Source: CAD feature listing. Evaluate the final solid. Frame: model axes, mm. Face numbers are marked on the shaded views. Coordinates: 2 decimals unless noted, no trailing zeros. Loops run counter-clockwise (first coordinate to the right, second up) from the corner with the lowest first, then second, coordinate; pieces in that order, holes last. Notation, with made-up numbers: (75, -30.5) - (86, -30.5) arc R20 cw to (86, -24.5) - close; hole circle Ø2 at (88, 46). An arc over 180 degrees is marked (long way). Write item = value, one per line. Start each with the question number.
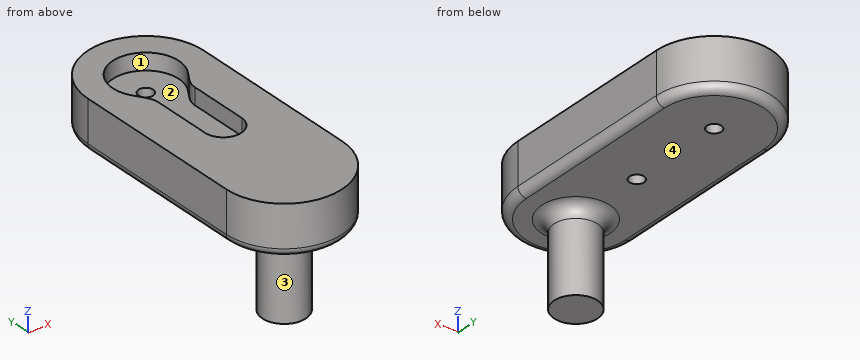
from build123d import *

# Parameters (mm, degrees)
PAD_DEPTH       = 12
POCKET_DEPTH    = 4
SKETCH002_R     = 5.25
PAD001_DEPTH    = 20
SKETCH003_R     = 1.75
POCKET001_DEPTH = 28.001
FILLET_R        = 3
FILLET001_R     = 2
FILLET002_R     = 5


with BuildPart() as part:
    # Sketch001 → Pad (new body)
    with BuildSketch(Plane.XY):
        with BuildLine():
            ThreePointArc((14, 0), (0, 14), (-14, 0))
            Line((-14, 0), (-14, -42))
            ThreePointArc((-14, -42), (0, -56), (14, -42))
            Line((14, -42), (14, 0))
        make_face()
    extrude(amount=PAD_DEPTH)

    # Sketch (on Face6 of Pad) → Pocket (cut)
    with BuildSketch(Plane.XY.offset(12)):
        with BuildLine():
            ThreePointArc((6.614378, -4.5), (0, 8), (-6.614378, -4.5))
            Line((-6.614378, -4.5), (-4.395452, -8))
            Line((-4.395452, -8), (-4.395452, -23.7))
            ThreePointArc((-4.395452, -23.7), (0, -27.9), (4.395452, -23.7))
            Line((4.395452, -8), (4.395452, -23.7))
            Line((6.614378, -4.5), (4.395452, -8))
        make_face()
    extrude(amount=-POCKET_DEPTH, mode=Mode.SUBTRACT)

    # Sketch002 (on Face4 of Pocket) → Pad001 (join)
    with BuildSketch(Plane(origin=(0, 0, 0), x_dir=(1, 0, 0), z_dir=(0, 0, -1))):
        with Locations((0, 42)):
            Circle(SKETCH002_R)
    extrude(amount=PAD001_DEPTH)

    # Sketch003 (on Face15 of Pad001) → Pocket001 (cut, through all)
    with BuildSketch(Plane.XY.offset(8)):
        Circle(SKETCH003_R)
        with Locations((0, -23.5)):
            Circle(SKETCH003_R)
    extrude(amount=-POCKET001_DEPTH, mode=Mode.SUBTRACT)

    # Fillet
    fillet_edges = [part.edges().sort_by_distance(p)[0] for p in [
        (-5.25, -42, 0),
    ]]
    fillet(fillet_edges, radius=FILLET_R)

    # Fillet001
    fillet001_edges = [part.edges().sort_by_distance(p)[0] for p in [
        (-14, -21, 0),
        (0, 14, 0),
        (14, -21, 0),
        (0, -56, 0),
    ]]
    fillet(fillet001_edges, radius=FILLET001_R)

    # Fillet002
    fillet002_edges = [part.edges().sort_by_distance(p)[0] for p in [
        (-4.395452, -8, 10),
        (4.395452, -8, 10),
    ]]
    fillet(fillet002_edges, radius=FILLET002_R)


solid = part.part
Item 1: Cut plane C-C (z = 3). Return the cut outline in (x, y).
Item 2: First-contact query: pin 1 (10 mm diameter, centred on x = 2, z = -7.5, fed in from +Y); pin 2 (3 mm diameter, centred on x = -1, y = -14, fed in from -Z); pin 3 (3 mm diameter, centred on x = 0, y = 0, fed in from +Z); pin 4 (9.5 mm diameter, centred on x = 0, y = 0, fed in from +Z). Flat tips, straight axial feed; report the tip coordinate or a pass-through.
Item 3: Draft query along X for the marked faces 1, 2, 3 and 4. Return one class per face: released by +X, released by -X, zero draft, split by the parting line, or undercut.
Item 4: Material intervals for L1, parallel to Y at x = 0, z = 2.5; L2, parallel to X at y = 0, z = 10; L3, parallel to Z at x = 3.75, y = -5.5, sorted ascending. Write a range as [from, to].
Item 5: Cut plane D-D (y = -29). Return the cut outline in (x, z).
Item 6: Cut plane B-B (y = -21). Return the cut outline in (x, z).
Item 7: Cut plane A-A (z = 9). Return the cut outline in (x, y).
Responses:
q1.outline = (-14, -42) arc R14 ccw to (14, -42) - (14, 0) arc R14 ccw to (-14, 0) - close; hole circle Ø3.5 at (0, -23.5); hole circle Ø3.5 at (0, 0)
q2.pin_1 = -36.75
q2.pin_2 = 0
q2.pin_3 = through
q2.pin_4 = 8
q3.face_1 = undercut
q3.face_2 = undercut
q3.face_3 = split by the parting line
q3.face_4 = zero draft
q4.L1 = [-56, -25.25], [-21.75, -1.75], [1.75, 14]
q4.L2 = [-14, -8], [8, 14]
q4.L3 = [0, 8]
q5.outline = (-14, 2) arc R2 ccw to (-12, 0) - (12, 0) arc R2 ccw to (14, 2) - (14, 12) - (-14, 12) - close
q6.outline = (-14, 2) arc R2 ccw to (-12, 0) - (12, 0) arc R2 ccw to (14, 2) - (14, 12) - (4.4, 12) - (4.4, 8) - (-4.4, 8) - (-4.4, 12) - (-14, 12) - close
q7.outline = (-14, -42) arc R14 ccw to (14, -42) - (14, 0) arc R14 ccw to (-14, 0) - close; hole (-6.61, -4.5) - (-5.17, -6.77) arc R5 cw to (-4.4, -9.45) - (-4.4, -23.7) arc R4.4 ccw to (4.4, -23.7) - (4.4, -9.45) arc R5 cw to (5.17, -6.77) - (6.61, -4.5) arc R8 ccw (long way) to start
